Design review of the part built by this model. Coordinates are the model's own, in mm. A direction names the side the tool comes from. Coordinates: 2 decimals unless noted, no trailing zeros. Loops run counter-clockwise (first coordinate to the right, second up) from the corner with the lowest first, then second, coordinate; pieces in that order, holes last. Notation, with made-up numbers: (-14, 66.5) - (29, 66.5) arc R25 cw to (29, 94.5) - close; hole circle Ø6 at (23.25, 86.25). An arc over 180 degrees is marked (long way). Answer in a Markdown table with one row per item. Add a question column.
(1) We need section C-C, the plane y = 14. Write out the cut boundary in (x, z), plus the area to 3 significant figures.
(2) Clearance check with flat-ended pins moving along their axes: pin 1 (5 mm diameter, centred on y = 21.5, z = 16.5, fed in from +X); pin 2 (1 mm diameter, centred on x = -27, z = 11.5, fed in from +Y); pin 3 (11 mm diameter, centred on x = -10, z = 22.5, fed in from +Y). State where each tip first meets the part, or that it passes through.
(3) To check wall thickness, follow L1, parallel to Y at x = -18.5, z = 8; L2, parallel to Z at x = -20, y = 36; L3, parallel to Z at x = -30, y = 38.5. State the ranges of each line that lie inside material, in increasing order. Write a range as [from, to].
(4) For faces 5 (the face through (-26, 34, 35)), 6 (the face through (-6, 9.818, 20)), 7 (the face through (-20, 15, 0)), list the 3-axis set-ups (+Z, -Z, +X, -X, +Y, -Y) from which the entire face can be reached by the end or side of a thin tool; tool diameter is ignored.
(5) The part is to be moulded in two halves that separate along Y. For faces 1 (the face through (-26, 37.068, 8)), 2 (the face through (-26, 40, 10)), 3 (the face through (-16, -3.182, 20)), 4 (the face through (-26, 32, 5)), say which applies: released by +Y, released by -Y, zero draft, split by the parting line, or undercut.
(6) We need section B-B, the plane z = 37. Write out the cut boundary in (x, y).
(7) We need section A-A, the plane x = -26. Write out the cut boundary in (y, z), plus the area to 3 significant figures.
(8) We need section D-D, the plane z = 31. Write out the cut boundary in (x, y).
from build123d import *

# Parameters (mm, degrees)
BOSS_EXTRUDE1_DEPTH = 40
SKETCH2_W           = 25
SKETCH2_H           = 5
CUT_EXTRUDE1_DEPTH  = 40
SKETCH3_W           = 30
SKETCH3_H           = 10.379013983
CUT_EXTRUDE2_DEPTH  = 40


with BuildPart() as part:
    # Sketch1 → Boss-Extrude1 (new body)
    with BuildSketch(Plane.XY):
        Polygon((-17.254373504, 42.068083371), (-35.254373504, 42.068083371), (-35.254373504, -3.181916629), (4.745626496, -3.181916629), (4.745626496, 9.818083371), (-17.254373504, 9.818083371), align=None)
    extrude(amount=BOSS_EXTRUDE1_DEPTH)

    # Sketch2 → Cut-Extrude1 (cut)
    with BuildSketch(Plane(origin=(-17.254373504, 0, 0), x_dir=(0, 0, -1), z_dir=(1, 0, 0))):
        with Locations((-22.5, 39.568083371)):
            Rectangle(SKETCH2_W, SKETCH2_H)
    extrude(amount=-CUT_EXTRUDE1_DEPTH, mode=Mode.SUBTRACT)

    # Sketch3 → Cut-Extrude2 (cut)
    with BuildSketch(Plane(origin=(-17.254373504, 0, 0), x_dir=(0, 0, -1), z_dir=(1, 0, 0))):
        with Locations((-20, 31.87857638)):
            Rectangle(SKETCH3_W, SKETCH3_H)
    extrude(amount=-CUT_EXTRUDE2_DEPTH, mode=Mode.SUBTRACT)


solid = part.part
Responses:
| question | item | result |
|---|---|---|
| 1 | outline | (-35.25, 0) - (-17.25, 0) - (-17.25, 40) - (-35.25, 40) - close |
| 1 | area | 720 mm2 |
| 2 | pin 1 | stops at x = -17.25 |
| 2 | pin 2 | stops at y = 26.69 |
| 2 | pin 3 | stops at y = 9.82 |
| 3 | L1 | y = [-3.18, 26.69], [37.07, 42.07] |
| 3 | L2 | z = [0, 5], [35, 40] |
| 3 | L3 | z = [0, 10], [35, 40] |
| 4 | face 5 | +X, -X, +Y |
| 4 | face 6 | +Z, -Z, +X, +Y |
| 4 | face 7 | -Z, +X, -X, +Y, -Y |
| 5 | face 1 | undercut |
| 5 | face 2 | zero draft |
| 5 | face 3 | released by -Y |
| 5 | face 4 | undercut |
| 6 | outline | (-35.25, -3.18) - (4.75, -3.18) - (4.75, 9.82) - (-17.25, 9.82) - (-17.25, 42.07) - (-35.25, 42.07) - close |
| 7 | outline | (-3.18, 0) - (42.07, 0) - (42.07, 10) - (37.07, 10) - (37.07, 5) - (26.69, 5) - (26.69, 35) - (42.07, 35) - (42.07, 40) - (-3.18, 40) - close |
| 7 | area | 1,370 mm2 |
| 8 | outline | (-35.25, -3.18) - (4.75, -3.18) - (4.75, 9.82) - (-17.25, 9.82) - (-17.25, 26.69) - (-35.25, 26.69) - close |
